```python
from build123d import *

# Parameters (mm, degrees)
SKETCH1_R           = 3
BOSS_EXTRUDE1_DEPTH = 35
SKETCH2_R           = 5.8
BOSS_EXTRUDE2_DEPTH = 4.3
FILLET1_R           = 1


with BuildPart() as part:
    # Sketch1 → Boss-Extrude1 (new body)
    with BuildSketch(Plane(origin=(0, 0, 0), x_dir=(1, 0, 0), z_dir=(0, 1, 0))):
        with Locations(Location((0, 0, 0), (0, 0, 270))):  # turned: the seam where the file's is
            Circle(SKETCH1_R)
    extrude(amount=BOSS_EXTRUDE1_DEPTH)

    # Sketch2 → Boss-Extrude2 (add)
    with BuildSketch(Plane(origin=(0, 35, 0), x_dir=(1, 0, 0), z_dir=(0, 1, 0))):
        with Locations(Location((0, 0, 0), (0, 0, 270))):  # turned: the seam where the file's is
            Circle(SKETCH2_R)
    extrude(amount=BOSS_EXTRUDE2_DEPTH)

    # Fillet1
    fillet1_edges = [part.edges().sort_by_distance(p)[0] for p in [
        (0, 35, -5.8),
        (0, 39.3, -5.8),
    ]]
    fillet(fillet1_edges, radius=FILLET1_R)


solid = part.part
```
Check sheet for the modelled part. Datum: model origin and axes. Units: mm. A direction names the side the tool comes from. Round coordinates to 2 decimals unless told otherwise and drop trailing zeros. Order: outer loops, then holes, each group sorted by start corner. A loop starts at its lowest first (then second) coordinate and runs counter-clockwise, first axis right, second up. Notation, with made-up numbers: (40.5, -24) -> (71.5, -24) arc R28 ccw to (71.5, 6) -> close; hole circle Ø5 at (-18.5, -28). An arc over 180 degrees is marked (long way). One line per item, written item: value. Start each with the question number.
Q1. Cross-section at C-C (y = 36.5). Record the boundary of the cut face in (x, z), and give its area (3 significant figures).
Q2. Thickness scan on line 1 (Y direction, x = 1.5, z = 4.5); line 2 (Y direction, x = -3.75, z = -3.75); line 3 (Z direction, x = 0.75, y = 4.5). Record the ranges inside material, lowest first.
Q3. Cross-section at B-B (z = 0). Record the boundary of the cut face in (x, y), and give its area (3 significant figures).
Q4. Gauge pin test, flat ends, axial feed: pin 1 Ø3 at (y, z) = (15.5, 1.5) entering from +X; pin 2 Ø5 at (x, z) = (-2.5, 1) entering from -Y; pin 3 Ø4 at (x, y) = (1.5, 27.5) entering from +Z; pin 4 Ø3 at (x, y) = (1.5, 34.5) entering from -Z. Record the tip position at first contact, or that the pin passes through.
Q5. Set-up check for faces 1 (the face through (0, 39.3, 0)), 2 (the face through (0.9, 17.26, 2.86)): record each of +Z, -Z, +X, -X, +Y, -Y from which the full face is reachable in a straight line by a thin tool's end or side.
Q6. Cross-section at D-D (y = 18). Record the boundary of the cut face in (x, z).
Q7. Cross-section at A-A (x = 0). Record the boundary of the cut face in (y, z).
Completed:
1. outline: circle Ø11.6 at (0, 0)
1. area: 106 mm²
2. line 1: y = 35 to 39.3
2. line 2: y = 35.14 to 39.16
2. line 3: z = -2.9 to 2.9
3. outline: (-5.8, 36) arc R1 ccw to (-4.8, 35) -> (-3, 35) -> (-3, 0) -> (3, 0) -> (3, 35) -> (4.8, 35) arc R1 ccw to (5.8, 36) -> (5.8, 38.3) arc R1 ccw to (4.8, 39.3) -> (-4.8, 39.3) arc R1 ccw to (-5.8, 38.3) -> close
3. area: 259 mm²
4. pin 1: stops at x = 3
4. pin 2: stops at y = 0
4. pin 3: stops at z = 3
4. pin 4: stops at z = -5.73
5. face 1: +Z, -Z, +X, -X, +Y
5. face 2: -Y
6. outline: circle Ø6 at (0, 0)
7. outline: (0, -3) -> (35, -3) -> (35, -4.8) arc R1 ccw to (36, -5.8) -> (38.3, -5.8) arc R1 ccw to (39.3, -4.8) -> (39.3, 4.8) arc R1 ccw to (38.3, 5.8) -> (36, 5.8) arc R1 ccw to (35, 4.8) -> (35, 3) -> (0, 3) -> close
